```python
from build123d import *

# Parameters (mm, degrees)
SKETCH1_W                = 153
SKETCH1_H                = 267
SKETCH1_W_2              = 77
SKETCH1_H_2              = 191
BOSS_EXTRUDE1_DEPTH      = 38
SKETCH2_W                = 38
SKETCH2_H                = 38
BOSS_EXTRUDE2_DEPTH      = 200
SKETCH3_W                = 38
SKETCH3_H                = 38
BOSS_EXTRUDE3_DEPTH      = 76.5
BOSS_EXTRUDE3_DEPTH_BACK = 76.5
BOSS_EXTRUDE4_DEPTH      = 38
SKETCH7_R                = 6.25
CUT_EXTRUDE1_DEPTH       = 154


with BuildPart() as part:
    # Sketch1 → Boss-Extrude1 (new body)
    with BuildSketch(Plane(origin=(0, 0, 0), x_dir=(1, 0, 0), z_dir=(0, 1, 0))):
        Rectangle(SKETCH1_W, SKETCH1_H)
        Rectangle(SKETCH1_W_2, SKETCH1_H_2, mode=Mode.SUBTRACT)
    extrude(amount=BOSS_EXTRUDE1_DEPTH)

    # Sketch2 → Boss-Extrude2 (add)
    with BuildSketch(Plane(origin=(0, 38, 0), x_dir=(1, 0, 0), z_dir=(0, 1, 0))):
        with Locations((0, 114.5)):
            Rectangle(SKETCH2_W, SKETCH2_H)
    extrude(amount=BOSS_EXTRUDE2_DEPTH)

    # Sketch3 → Boss-Extrude3 (add, two sides)
    with BuildSketch(Plane(origin=(0, 0, 0), x_dir=(0, 0, -1), z_dir=(1, 0, 0))) as boss_extrude3_sk:
        with Locations((114.5, 257)):
            Rectangle(SKETCH3_W, SKETCH3_H)
    extrude(amount=BOSS_EXTRUDE3_DEPTH)
    extrude(boss_extrude3_sk.sketch, amount=-BOSS_EXTRUDE3_DEPTH_BACK)

    # Sketch6 → Boss-Extrude4 (add)
    with BuildSketch(Plane(origin=(76.5, 0, 0), x_dir=(0, 0, -1), z_dir=(1, 0, 0))):
        Polygon((95.5, 276), (-81.5, 38), (-34.143309895, 38), (114.596185904, 238), (95.5, 238), align=None)
    boss_extrude4 = extrude(amount=-BOSS_EXTRUDE4_DEPTH)

    # Mirror1: Boss-Extrude4 across plane
    add(boss_extrude4.mirror(Plane(origin=(0, 0, 0), x_dir=(0, 0, 1), z_dir=(1, 0, 0))))

    # Sketch7 → Cut-Extrude1 (cut, through all)
    with BuildSketch(Plane(origin=(76.5, 0, 0), x_dir=(0, 0, -1), z_dir=(1, 0, 0))):
        with Locations((57.5, 19)):
            Circle(SKETCH7_R)
    extrude(amount=-CUT_EXTRUDE1_DEPTH, mode=Mode.SUBTRACT)


solid = part.part
```
Can you work these out from the model? Positions are in its coordinate system, mm. A direction names the side the tool comes from. Coordinates: 2 decimals unless noted, no trailing zeros. Loops run counter-clockwise (first coordinate to the right, second up) from the corner with the lowest first, then second, coordinate; pieces in that order, holes last.
1) Imagine slicing it at B-B on y = 19. List the corners of the cut face in (x, z) for me, plus the area to 3 significant figures.
2) Imagine slicing it at A-A on x = -2. List the corners of the cut face in (y, z) for me, plus the area to 3 significant figures.
3) I need wall thicknesses on probe 1 along X at (y, z) = (118, 10); probe 2 along Y at (x, z) = (59, -57); probe 3 along Y at (x, z) = (-68, -57.5). Which ranges of each line are inside material? Lowest first, please.
4) Imagine slicing it at D-D on z = -57.5. List the corners of the cut face in (x, y) for me, plus the area to 3 significant figures.
5) Thinking about a two-plate mould opening in Y: for faces 1 (the flat face through (76.5, 98, -9)), 2 (the flat face through (19, 137, -114)), 3 (the flat face through (1, 276, -114)), which applies, pulls with the +Y half, pulls with the -Y half, needs draft (parallel to the pull), parting line crosses it, or undercut?
6) Which directions (+Z, -Z, +X, -X, +Y, -Y) give clear straight access to the entire face, cutting with the end or side of a thin tool? Please do faces 4 (the flat face through (-76.5, 98, -9)), 5 (the flat face through (-41, 238, -118)), 6 (the flat face through (-1, 38, 107)), 7 (the flat face through (-55, 38, -51)), 8 (the cylindrical face through (57.766, 16.606, -63.273)).
7) For pin 1 (4 mm diameter, centred on x = -37, y = 83.5, fed in from -Z); pin 2 (5 mm diameter, centred on x = -34.5, z = -41, fed in from -Y), each with a flat end and sliding along its axis, tell me the tip position at first contact or that it passes through.
8) Imagine slicing it at C-C on x = 31.5. List the corners of the cut face in (y, z) for me, plus the area to 3 significant figures.
Completed:
1. outline: (-76.5, -133.5) - (76.5, -133.5) - (76.5, -63.75) - (38.5, -63.75) - (38.5, -95.5) - (-38.5, -95.5) - (-38.5, -63.75) - (-76.5, -63.75) - close; (-76.5, -51.25) - (-38.5, -51.25) - (-38.5, 95.5) - (38.5, 95.5) - (38.5, -51.25) - (76.5, -51.25) - (76.5, 133.5) - (-76.5, 133.5) - close
1. area: 25,200 mm2
2. outline: (0, -133.5) - (276, -133.5) - (276, -95.5) - (0, -95.5) - close; (0, 95.5) - (38, 95.5) - (38, 133.5) - (0, 133.5) - close
2. area: 11,900 mm2
3. probe 1: x = -76.5 to -38.5, 38.5 to 76.5
3. probe 2: y = 0 to 12.77, 25.23 to 38, 160.55 to 224.23
3. probe 3: y = 0 to 12.75, 25.25 to 38, 161.23 to 224.9
4. outline: (-76.5, 0) - (-38.5, 0) - (-38.5, 12.75) - (-76.5, 12.75) - close; (-76.5, 25.25) - (-38.5, 25.25) - (-38.5, 38) - (-76.5, 38) - close; (-76.5, 161.23) - (-38.5, 161.23) - (-38.5, 224.9) - (-76.5, 224.9) - close; (38.5, 0) - (76.5, 0) - (76.5, 12.75) - (38.5, 12.75) - close; (38.5, 25.25) - (76.5, 25.25) - (76.5, 38) - (38.5, 38) - close; (38.5, 161.23) - (76.5, 161.23) - (76.5, 224.9) - (38.5, 224.9) - close
4. area: 6,780 mm2
5. face 1: needs draft
5. face 2: undercut
5. face 3: pulls with the +Y half
6. face 4: +Z, -Z, -X, +Y, -Y
6. face 5: -Z
6. face 6: +Z, +X, -X, +Y
6. face 7: -Z, -X
6. face 8: +X, -X
7. pin 1: stops at z = -0.68
7. pin 2: passes through
8. outline: (0, -133.5) - (38, -133.5) - (38, -95.5) - (0, -95.5) - close; (0, 95.5) - (38, 95.5) - (38, 133.5) - (0, 133.5) - close; (238, -133.5) - (276, -133.5) - (276, -95.5) - (238, -95.5) - close
8. area: 4,330 mm2
